Source: CAD feature listing. Evaluate the final solid. Frame: model axes, mm. Face numbers are marked on the shaded views. A direction names the side the tool comes from. Coordinates: 2 decimals unless noted, no trailing zeros. Write each loop counter-clockwise with the first axis right and the second up, starting at its lowest first coordinate (ties: lowest second). Pieces come first, ordered by that corner, then holes. Notation, with made-up numbers: (28, 72.25) - (61, 72.25) arc R19 ccw to (61, 102.25) - close; hole circle Ø6 at (-8, 46.5). An arc over 180 degrees is marked (long way). One line per question, with ' | ' between items.
from build123d import *

# Parameters (mm, degrees)
F0_W       = 114.3609508872
F0_H       = 162.4245643616
F1_DEPTH   = 25.4
F2_W       = 114.3609508872
F2_H       = 32.8328199685
F2_H_2     = 27.7516581118
F3_DEPTH   = 101.6
F4_R       = 21.0436715378
F3_FACE1_W = 114.3609508872
F3_FACE1_H = 101.6
F5_DEPTH   = 228.6
F6_R       = 33.8173420759
F6_R_2     = 21.0436715378
F10_DEPTH  = 12.7
F9_R       = 35.2124743409
F9_R_2     = 21.0436715378
F11_DEPTH  = 12.7
F12_R      = 5.08
F7_R       = 37.8739843542
F7_R_2     = 21.0436715378
F13_DEPTH  = 12.7
F8_R       = 36.6649491414
F8_R_2     = 21.0436715378
F14_DEPTH  = 12.7
F15_R      = 12.7


with BuildPart() as f1:
    # F0 (on Front) → F1 (new body)
    with BuildSketch(Plane.XZ):
        Rectangle(F0_W, F0_H)
    extrude(amount=F1_DEPTH)

    # F2 (on face) → F3 (join)
    with BuildSketch(Plane.XZ.offset(25.4)):
        with Locations((0, 32.0948231965)):
            Rectangle(F2_W, F2_H)
        with Locations((0, -32.6631646603)):
            Rectangle(F2_W, F2_H_2)
    extrude(amount=F3_DEPTH)

    # F4 (on face) + F3_face1 (on face) → F5 (cut)
    with BuildSketch(Plane.XY.offset(48.5112331808)):
        with Locations((0, -84.3189582229)):
            Circle(F4_R)
    with BuildSketch(Plane(origin=(0, -76.2, -46.5389937162), x_dir=(1, 0, 0), z_dir=(0, 0, -1))):
        Rectangle(F3_FACE1_W, F3_FACE1_H)
    extrude(amount=-F5_DEPTH, dir=(0, 0, 1), mode=Mode.SUBTRACT)

    # F6 (on face) → F10 (join)
    with BuildSketch(Plane.XY.offset(48.5112331808)):
        with Locations((0, -84.3189582229)):
            Circle(F6_R)
        with Locations((0, -84.3189582229)):
            Circle(F6_R_2, mode=Mode.SUBTRACT)
    extrude(amount=F10_DEPTH)

    # F9 (on face) → F11 (join)
    with BuildSketch(Plane(origin=(0, 0, -46.5389937162), x_dir=(1, 0, 0), z_dir=(0, 0, -1))):
        with Locations((0, 84.3189582229)):
            Circle(F9_R)
        with Locations((0, 84.3189582229)):
            Circle(F9_R_2, mode=Mode.SUBTRACT)
    extrude(amount=F11_DEPTH)

    # F12
    f12_edges = [f1.edges().sort_by_distance(p)[0] for p in [
        (0, -25.4, 48.511233),
        (0, -25.4, 15.678413),
        (0, -25.4, -18.787336),
        (0, -25.4, -46.538994),
    ]]
    fillet(f12_edges, radius=F12_R)

    # F7 (on face) → F13 (join)
    with BuildSketch(Plane(origin=(0, 0, 15.6784132123), x_dir=(1, 0, 0), z_dir=(0, 0, -1))):
        with Locations((0, 84.3189582229)):
            Circle(F7_R)
        with Locations((0, 84.3189582229)):
            Circle(F7_R_2, mode=Mode.SUBTRACT)
    extrude(amount=F13_DEPTH)

    # F8 (on face) → F14 (join)
    with BuildSketch(Plane.XY.offset(-18.7873356044)):
        with Locations((0, -84.3189582229)):
            Circle(F8_R)
        with Locations((0, -84.3189582229)):
            Circle(F8_R_2, mode=Mode.SUBTRACT)
    extrude(amount=F14_DEPTH)

    # F15
    f15_edges = [f1.edges().sort_by_distance(p)[0] for p in [
        (57.180475, -127, -32.663165),
        (57.180475, -127, 32.094823),
        (-57.180475, -127, -32.663165),
        (-57.180475, -127, 32.094823),
    ]]
    fillet(f15_edges, radius=F15_R)


solid = f1.part
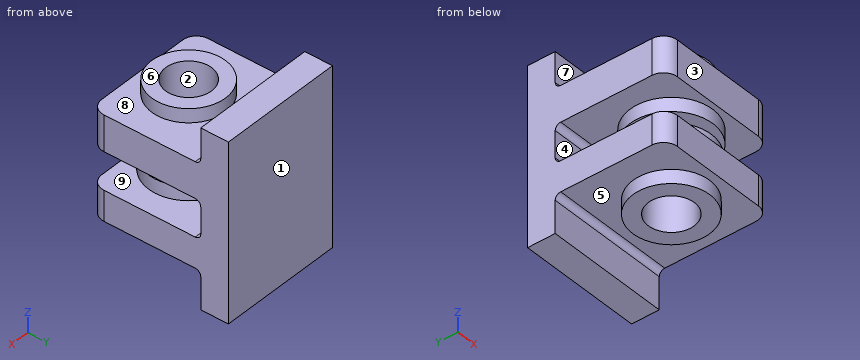
Item 1: Cut plane D-D on x = 0. State how many separate pieces and enclosed holes the cut face has, and give its area (3 significant figures).
Check sheet entries:
separate pieces: 3 | enclosed holes: 0 | area: 9,260 mm²
Item 2: Pin query (flat end, axial travel): pin 1 Ø12 at (x, y) = (42, -37) entering from +Z; pin 2 Ø1.5 at (x, y) = (14.5, -45) entering from -Z; pin 3 Ø8 at (x, y) = (20.5, -105.5) entering from -Z. Return the tip coordinate at first contact, or that it passes through.
Check sheet entries:
pin 1: z = 48.51 | pin 2: z = -46.54 | pin 3: z = -59.24
Item 3: Access query for the marked faces 5, 6, 7, 8 and 9. Directions: +Z, -Z, +X, -X, +Y, -Y. A direction counts if a zero-diameter tool reaches every point of the face in a straight line with its end or side. Return the directions, or none.
Check sheet entries:
face 5: -Z | face 6: +Z, +X, -X, -Y | face 7: +Z, +X, -X | face 8: +Z | face 9: none
Item 4: Cut plane B-B on y = -110. Return loops of the section in (x, z), and give its area (3 significant figures).
Check sheet entries:
outline: (-57.18, -46.54) - (-24.09, -46.54) - (-24.09, -59.24) - (24.09, -59.24) - (24.09, -46.54) - (57.18, -46.54) - (57.18, -18.79) - (26.17, -18.79) - (26.17, -6.09) - (-26.17, -6.09) - (-26.17, -18.79) - (-57.18, -18.79) - close; (-57.18, 15.68) - (-27.84, 15.68) - (-27.84, 2.98) - (27.84, 2.98) - (27.84, 15.68) - (57.18, 15.68) - (57.18, 48.51) - (22, 48.51) - (22, 61.21) - (-22, 61.21) - (-22, 48.51) - (-57.18, 48.51) - close | area: 9,470 mm²
Item 5: Mould query, pull axis Y, two halves, no side actions, for the marked faces 1, 2, 3 and 4. Classes: pulls with the +Y half, pulls with the -Y half, needs draft (parallel to the pull), parting line crosses it, or undercut.
Check sheet entries:
face 1: pulls with the +Y half | face 2: undercut | face 3: pulls with the -Y half | face 4: undercut
Item 6: Ray query, line 1 along Z through (x, y) = (-20.5, -31.5); line 2 along Z through (x, y) = (-10.5, -106); line 3 along Y through (x, z) = (0, -21). Return the intervals inside material, ascending. Write a range as [from, to].
Check sheet entries:
line 1: [-46.54, -18.79], [15.68, 48.51] | line 2: [-59.24, -6.09], [2.98, 61.21] | line 3: [-127, -105.36], [-63.28, 0]
Item 7: Cut plane A-A on z = 21. Return loops of the section in (x, y).
Check sheet entries:
outline: (-57.18, -114.3) arc R12.7 ccw to (-44.48, -127) - (44.48, -127) arc R12.7 ccw to (57.18, -114.3) - (57.18, 0) - (-57.18, 0) - close; hole circle Ø42.09 at (0, -84.32)
